from build123d import *

# Parameters (mm, degrees)
MASTER_SKETCH_WING_GEOMETRY_MASTER_SKETC_R   = 10
MASTER_SKETCH_WING_GEOMETRY_MASTER_SKETC_W   = 92
MASTER_SKETCH_WING_GEOMETRY_MASTER_SKETC_H   = 38
MASTER_SKETCH_WING_GEOMETRY_MASTER_SKETC_R_2 = 12.5
MASTER_SKETCH_WING_GEOMETRY_MASTER_SKETC_R_3 = 17.5
BOSS_EXTRUDE2_DEPTH                          = 5


with BuildPart() as part:
    # Master sketch-Wing Geometry Master Sketc → Boss-Extrude2 (new body)
    with BuildSketch(Plane.XY):
        with BuildLine():
            Line((210.07475011, 20.55043194), (211.114806417, 25.441064095))
            add(Edge.make_bspline(
                [(211.114806417, 25.441064095), (210.423359837, 25.588109171), (208.256226378, 26.046518307), (204.590060504, 26.80992466), (200.100470305, 27.709491549), (195.551555784, 28.574874953), (190.957101153, 29.440580512), (186.312819207, 30.266153712), (181.629850434, 31.069092462), (176.911633472, 31.833504414), (172.163553808, 32.589756341), (167.386378314, 33.297913229), (162.585397476, 33.965141895), (157.772606773, 34.60690524), (152.945783838, 35.207030951), (148.116103717, 35.768371218), (143.281947921, 36.275964114), (138.451826021, 36.746166863), (133.632024585, 37.177420244), (128.825099136, 37.557009572), (124.035268277, 37.890964919), (119.227934324, 38.158056396), (114.414879536, 38.383930966), (109.600810746, 38.523171189), (104.830170116, 38.581209103), (100.103024464, 38.571187104), (95.428917776, 38.495242632), (90.811807971, 38.332326352), (86.257821528, 38.103740215), (81.770642032, 37.802892678), (77.355663903, 37.439401702), (73.023107372, 36.981755849), (68.77458737, 36.478522782), (64.618104025, 35.895217538), (60.552867783, 35.25916861), (56.589427231, 34.548268384), (52.728147609, 33.780528228), (48.978480985, 32.948622201), (45.340648206, 32.070500948), (41.817597831, 31.144685204), (38.422513869, 30.152277869), (35.148426276, 29.122139824), (32.002488884, 28.056760571), (28.991053216, 26.94735735), (26.116143259, 25.797761949), (23.382030001, 24.605992477), (21.092241599, 23.54817715), (19.726805869, 22.866225277), (19.219088354, 22.606550883)],
                knots=[0.147831525, 0.147831525, 0.147831525, 0.147831525, 0.151223285, 0.15845953, 0.165799086, 0.173192204, 0.180676633, 0.188231103, 0.195824579, 0.203473251, 0.211164227, 0.218892942, 0.226644195, 0.234420668, 0.24218898, 0.249981423, 0.257749175, 0.26551047, 0.273265831, 0.280966678, 0.288645672, 0.296302699, 0.304067471, 0.31176355, 0.319408994, 0.326957892, 0.334443893, 0.34183727, 0.349123554, 0.356320599, 0.363414403, 0.370376839, 0.377222796, 0.383940401, 0.390513899, 0.396964017, 0.403259098, 0.409401768, 0.415391075, 0.421213922, 0.426877502, 0.432360647, 0.437681281, 0.442812195, 0.447757077, 0.452534713, 0.457121248, 0.459857253, 0.459857253, 0.459857253, 0.459857253], degree=3))
            Line((19.219088354, 22.606550883), (21.49585547, 18.154997053))
            add(Edge.make_bspline(
                [(21.49585547, 18.154997053), (-12.082056869, 0.079644189), (21.495939944, -8.707202746)],
                knots=[0, 0, 0, 1, 1, 1], degree=2))
            Line((21.495939944, -8.707202746), (20.394317181, -13.584335848))
            add(Edge.make_bspline(
                [(20.394317181, -13.584335848), (20.878636368, -13.693731476), (22.176487001, -13.975597653), (24.333802223, -14.388616706), (26.902677481, -14.802759919), (29.579032983, -15.186644107), (32.364727066, -15.507317142), (35.24979682, -15.818395551), (38.24224316, -16.045446189), (41.331828524, -16.260981777), (44.519015875, -16.42830612), (47.799283263, -16.558119697), (51.16623897, -16.647932894), (54.61986093, -16.695073811), (58.159965351, -16.714295991), (61.783518843, -16.708264717), (65.483463359, -16.650825987), (69.256985649, -16.584892049), (73.10377458, -16.484484885), (77.020259272, -16.35080262), (81.003979497, -16.205643438), (85.050068364, -16.018089633), (89.157165379, -15.833715938), (93.320145134, -15.619391907), (97.536821023, -15.399674924), (101.807253217, -15.173788761), (106.123150678, -14.916806976), (110.483633277, -14.67183184), (114.883266318, -14.40885373), (119.352975093, -14.1438502), (123.894349232, -13.897019305), (128.496857287, -13.599501008), (133.130234778, -13.300324022), (137.784055517, -12.993867357), (142.453682427, -12.661474057), (147.129863453, -12.318169381), (151.814228379, -11.985316734), (156.499893797, -11.618572445), (161.183377828, -11.260601924), (165.86046019, -10.90254886), (170.523341726, -10.530097392), (175.17012114, -10.161520293), (179.793367843, -9.790428778), (184.3901672, -9.422077018), (188.959593481, -9.048259618), (193.49686261, -8.692457096), (197.993446272, -8.331402015), (202.443627904, -7.973643055), (206.497194094, -7.635119669), (209.069001496, -7.436255041), (210.173597999, -7.350571372)],
                knots=[0.551686861, 0.551686861, 0.551686861, 0.551686861, 0.554069096, 0.558058927, 0.562223755, 0.566552856, 0.571030235, 0.575677162, 0.580474566, 0.585427924, 0.590537056, 0.595787007, 0.601178702, 0.606697002, 0.612358753, 0.618164376, 0.624082472, 0.63011302, 0.636272552, 0.642545409, 0.648915298, 0.655399016, 0.66197932, 0.668641043, 0.67539942, 0.682238498, 0.689159203, 0.696143776, 0.703193144, 0.710306375, 0.717627174, 0.725014702, 0.73243517, 0.739904564, 0.747392102, 0.754896736, 0.762401371, 0.769924336, 0.777447302, 0.784938376, 0.792430695, 0.799891129, 0.807303734, 0.814684455, 0.822017351, 0.829301143, 0.836521163, 0.843661474, 0.850722081, 0.856037867, 0.856037867, 0.856037867, 0.856037867], degree=3))
            Line((210.173597999, -7.350571372), (209.78690169, -2.365451127))
            Line((209.78690169, -2.365451127), (219.93, -1.558186688))
            Line((219.93, -1.558186688), (219.93, 18.391622486))
            Line((219.93, 18.391622486), (210.07475011, 20.55043194))
        make_face()
        with Locations((26.291015868, 4.759044754)):
            Circle(MASTER_SKETCH_WING_GEOMETRY_MASTER_SKETC_R, mode=Mode.SUBTRACT)
        with Locations((90.000000001, 9.799999997)):
            Rectangle(MASTER_SKETCH_WING_GEOMETRY_MASTER_SKETC_W, MASTER_SKETCH_WING_GEOMETRY_MASTER_SKETC_H, mode=Mode.SUBTRACT)
        with Locations((195.809022747, 9.888215346)):
            Circle(MASTER_SKETCH_WING_GEOMETRY_MASTER_SKETC_R_2, mode=Mode.SUBTRACT)
        with Locations((159.205482831, 11.38801065)):
            Circle(MASTER_SKETCH_WING_GEOMETRY_MASTER_SKETC_R_3, mode=Mode.SUBTRACT)
    extrude(amount=BOSS_EXTRUDE2_DEPTH)


solid = part.part
CAD build for the part. Positions are in the model's coordinates, mm. A direction names the side the tool comes from. Give positions to 0.01 mm unless a question says otherwise; leave off trailing zeros. Return JSON: item names as keys, results as strings.
Item 1: Tool access for faces 1 (the flat face through (89, 28.8, 2)), 2 (the flat face through (20.953, -11.112, 2.465)), 3 (the flat face through (210.587, 22.962, 2.465)): list every direction of +Z, -Z, +X, -X, +Y, -Y with a clear straight run to the whole face (end or side of a thin tool).
Answer below:
{"face 1": "+Z, -Z", "face 2": "+Z, -Z, -X", "face 3": "+Z, -Z, +X"}
Item 2: Drill centre lines: probe 1 along X at (y, z) = (21.5, 1.6); probe 2 along X at (y, z) = (5.5, 2.45); probe 3 along X at (y, z) = (13.5, 4.7). Where is each one in solid material? Low to high.
Answer below:
{"probe 1": "x = 19.79 to 44, 136 to 144.92, 173.49 to 191.18, 200.44 to 210.28", "probe 2": "x = 5.54 to 16.32, 36.26 to 44, 136 to 142.73, 175.69 to 184.1, 207.51 to 219.93", "probe 3": "x = 13.74 to 21.43, 31.15 to 44, 136 to 141.83, 176.58 to 183.84, 207.78 to 219.93"}
Item 3: Band-saw the part on A-A (z = 3.6). Give the number of separate pieces and of enclosed holes in the cut face, then the cut area to 3 significant figures.
Answer below:
{"separate pieces": "1", "enclosed holes": "4", "area": "4,200 mm2"}
Item 4: Two-plate mould, pull along X, no slides. Class faces 4 (the flat face through (136, 10, 2)), 5 (the flat face through (209.983, -4.893, 2.465)), 6 (the flat face through (120.6, -9.4, 5)): +X half, -X half, draft (parallel to the pull), parting line (faces both ways), or undercut.
Answer below:
{"face 4": "undercut", "face 5": "+X half", "face 6": "draft"}
Item 5: Drop flat-ended pins along their axis: pin 1 (1.5 mm diameter, centred on x = 43.5, z = 3.5, fed in from +Y); pin 2 (22.5 mm diameter, centred on x = 195.81, y = 9.89, fed in from +Z); pin 3 (2.5 mm diameter, centred on y = 16.5, z = 2.5, fed in from -X). Give the stop position or say it passes through.
Answer below:
{"pin 1": "stops at y = 31.78", "pin 2": "passes through", "pin 3": "stops at x = 16.44"}
